```python
from build123d import *

# Parameters (mm, degrees)
CYLINDER003_R     = 2
CYLINDER003_DEPTH = 10
CYLINDER001_R     = 2
CYLINDER001_DEPTH = 10
SKETCH037_W       = 7.5
SKETCH037_H       = 7.5
EXTRUDE045_DEPTH  = 10
SKETCH005_R       = 1.3
EXTRUDE003_DEPTH  = 20
EXTRUDE039_DEPTH  = 4
EXTRUDE042_DEPTH  = 0.8
EXTRUDE002_DEPTH  = 6
EXTRUDE037_DEPTH  = 2


with BuildPart() as shutter_cable001:
    # Cylinder003 → Cylinder003 (new body)
    with BuildSketch(Plane(origin=(19.5, 0, 24.5), x_dir=(1, 0, 0), z_dir=(0, 0, 1))):
        Circle(CYLINDER003_R)
    extrude(amount=CYLINDER003_DEPTH)


with BuildPart() as battery_cable:
    # Cylinder001 → Cylinder001 (new body)
    with BuildSketch(Plane(origin=(-70.5, 0, 12), x_dir=(0, 0, 1), z_dir=(-1, 0, 0))):
        Circle(CYLINDER001_R)
    extrude(amount=CYLINDER001_DEPTH)


with BuildPart() as common_sub:
    # Sketch037 → Extrude045 (new body)
    with BuildSketch(Plane.YZ.offset(35)):
        with Locations((0, 12)):
            Rectangle(SKETCH037_W, SKETCH037_H)
    extrude(amount=EXTRUDE045_DEPTH)


with BuildPart() as common_sub_1:
    # Extrude045 placement: moved
    add(common_sub.part.moved(Location((-9.5, 0, 0))))

    # Fusion033: union shutter cable001, battery cable
    add(shutter_cable001.part)
    add(battery_cable.part)


with BuildPart() as sweep001:
    # Sweep001: sweep along a path in Sketch034
    with BuildLine(Plane.XZ.offset(10)) as sweep001_path:
        Line((32, 12), (32, 26.4))
        ThreePointArc((32, 26.4), (30.652691, 29.652691), (27.4, 31))
        Line((27.4, 31), (-39.9, 31))
    # Sketch035 → Sweep001 (sweep)
    with BuildSketch(Plane.YZ):
        Polygon((5.3, 29.4), (3.7, 31), (3.7, 32), (6, 32), (6, 29.4), align=None)
    sweep(path=sweep001_path.line)


with BuildPart() as fusion030:
    # Sketch005 → Extrude003 (new body)
    with BuildSketch(Plane.XZ.offset(5)):
        with Locations((27.4, 26.4)):
            Circle(SKETCH005_R)
    extrude(amount=-EXTRUDE003_DEPTH)


with BuildPart() as fusion030_1:
    # Extrude003 placement: moved
    add(fusion030.part.moved(Location((0, -4, 0))))

    # Fusion030: union Sweep001
    add(sweep001.part)


with BuildPart() as top003:
    # Sketch028 → Extrude039 (new body)
    with BuildSketch(Plane.XZ.offset(10)):
        with BuildLine():
            ThreePointArc((32, 26.4), (30.652691, 29.652691), (27.4, 31))
            Line((27.4, 31), (-39.9, 31))
            Line((-39.9, 31), (-39.9, 29))
            Line((-39.9, 29), (27.4, 29))
            ThreePointArc((30, 26.4), (29.238478, 28.238478), (27.4, 29))
            Line((30, 12), (30, 26.4))
            Line((32, 12), (30, 12))
            Line((32, 26.4), (32, 12))
        make_face()
    extrude(amount=EXTRUDE039_DEPTH)


with BuildPart() as top003_1:
    # Extrude039 placement: moved
    add(top003.part.moved(Location((0, 14.5, 0))))


with BuildPart() as top002:
    # Sketch031 → Extrude042 (new body)
    with BuildSketch(Plane.XZ.offset(10)):
        with BuildLine():
            ThreePointArc((32, 26.4), (30.652691, 29.652691), (27.4, 31))
            Line((27.4, 31), (-39.9, 31))
            Line((-39.9, 31), (-39.9, 12))
            Line((-39.9, 12), (32, 12))
            Line((32, 26.4), (32, 12))
        make_face()
    extrude(amount=EXTRUDE042_DEPTH)


with BuildPart() as top002_1:
    # Extrude042 placement: moved
    add(top002.part.moved(Location((0, 15.3, 0))))


with BuildPart() as screw_hole_top:
    # Sketch004 → Extrude002 (new body)
    with BuildSketch(Plane.XZ.offset(10)):
        with BuildLine():
            ThreePointArc((25.36776, 29), (25.066548, 24.066548), (30, 24.36776))
            Line((30, 24.36776), (30, 26.4))
            ThreePointArc((30, 26.4), (29.238478, 28.238478), (27.4, 29))
            Line((25.36776, 29), (27.4, 29))
        make_face()
    extrude(amount=-EXTRUDE002_DEPTH)


with BuildPart() as screw_hole_top_1:
    # Extrude002 placement: moved
    add(screw_hole_top.part.moved(Location((0, 8.5, 0))))


with BuildPart() as top:
    # Sketch029 → Extrude037 (new body)
    with BuildSketch(Plane.XZ.offset(10)):
        with BuildLine():
            ThreePointArc((30.9, 26.4), (29.874874, 28.874874), (27.4, 29.9))
            Line((27.4, 29.9), (-22.5, 29.9))
            Line((-22.5, 29.9), (-22.5, 29))
            Line((-22.5, 29), (27.4, 29))
            ThreePointArc((30, 26.4), (29.238478, 28.238478), (27.4, 29))
            Line((30, 12), (30, 26.4))
            Line((30.9, 12), (30, 12))
            Line((30.9, 26.4), (30.9, 12))
        make_face()
    extrude(amount=EXTRUDE037_DEPTH)


with BuildPart() as top_1:
    # Extrude037 placement: moved
    add(top.part.moved(Location((0, 10.5, 0))))

    # Fusion028: union top003, top002, screw hole top
    add(top003_1.part)
    add(top002_1.part)
    add(screw_hole_top_1.part)

    # Cut024: cut Fusion030
    add(fusion030_1.part, mode=Mode.SUBTRACT)


with BuildPart() as part_mirroring:
    # Part__Mirroring: instance of top
    add(top_1.part.mirror(Plane(origin=(0, 0, 12), x_dir=(0, 1, 0), z_dir=(0, 0, 1))))


with BuildPart() as part_mirroring002:
    # Part__Mirroring002: instance of Part__Mirroring
    add(part_mirroring.part.mirror(Plane(origin=(-22.5, 1, 0), x_dir=(0, -1, 0), z_dir=(1, 0, 0))))


with BuildPart() as top007:
    # Part__Mirroring003: instance of top
    add(top_1.part.mirror(Plane(origin=(-22.5, 0, 0), x_dir=(0, -1, 0), z_dir=(1, 0, 0))))

    # Fusion032: union top, Part__Mirroring, Part__Mirroring002
    add(top_1.part)
    add(part_mirroring.part)
    add(part_mirroring002.part)

    # Cut025: cut common sub
    add(common_sub_1.part, mode=Mode.SUBTRACT)


solid = top007.part
```
Can you work these out from the model? Positions are in its coordinate system, mm. A direction names the side the tool comes from. Coordinates: 2 decimals unless noted, no trailing zeros. Write each loop counter-clockwise with the first axis right and the second up, starting at its lowest first coordinate (ties: lowest second). Pieces come first, ordered by that corner, then holes. Notation, with made-up numbers: M 60.5,21 L 78.5,21 A14 cw 78.5,45 Z; hole C 50,1.5 d7. An arc over 180 degrees is marked long. Write item = value, one per line. Start each with the question number.
Q1. If I drill on L1, parallel to Z at x = -72.4, y = 3.5; L2, parallel to Z at x = -65.5, y = -1; L3, parallel to X at y = 1.5, z = 25.5, over which ranges is the centre line in solid material (lowest first)? Write a range as [from, to].
Q2. I'm going to push flat-ended pins straight in: pin 1 (0.6 mm diameter, centred on y = -1, z = 21.5, fed in from -X); pin 2 (0.6 mm diameter, centred on x = 30.5, y = 2, fed in from -Z); pin 3 (1 mm diameter, centred on x = -12, y = 4.5, fed in from +Z). Where does each tip first touch, or does it pass through?
Q3. If we section it at C-C, the plane z = 12: Write out the boundary of the cut face in (x, y), then the cut area to 3 significant figures.
Q4. If we section it at B-B, the plane x = -58: Write out the boundary of the cut face in (y, z), then the cut area to 3 significant figures.
Q5. On a 3-axis mill with a long thin cutter (end or side, diameter ignored), from which of +Z, -Z, +X, -X, +Y, -Y can I reach the whole of each face in a straight line? I mean faces 1 (the face through (-74.9, -0.49, 28.85)), 2 (the face through (-75.9, 0, 20)), 3 (the face through (-22, 2, -5)). Say none if no direction works.
Q6. Thinking about a two-plate mould opening in Z: for faces 4 (the face through (31, 3.75, 12)), 5 (the face through (-71.1, 1.85, -2.46)), 6 (the face through (-23, 2, -7)), 7 (the face through (30.9, 0, 3)), which applies, released by +Z, released by -Z, zero draft, split by the parting line, or undercut?
Q7. If we section it at A-A, the plane z = 21.5: Write out the boundary of the cut face in (x, y), then the cut area to 3 significant figures.
Check sheet entries:
q1.L1 = [-7, -3.7], [-1.1, 0.9], [23.1, 25.1], [27.7, 31]
q1.L2 = [-5.9, -5], [29, 29.9]
q1.L3 = [-77, -73.34], [-71.46, -69.23], [24.23, 26.46], [28.34, 32]
q2.pin_1 = -75.9
q2.pin_2 = -6.05
q2.pin_3 = 30.7
q3.outline = M -77,2 L -75,2 L -75,4.5 L 30,4.5 L 30,3.75 L 31.95,3.75 L 30.4,5.3 L -75.4,5.3 L -77,3.7 Z
q3.area = 91.1 mm²
q4.outline = M -1.5,-5.9 L 0.5,-5.9 L 0.5,-7 L 3.7,-7 L 5.3,-5.4 L 5.3,29.4 L 3.7,31 L 0.5,31 L 0.5,29.9 L -1.5,29.9 L -1.5,29 L 4.5,29 L 4.5,-5 L -1.5,-5 Z
q4.area = 47.4 mm²
q5.face_1 = +Z, -X, -Y
q5.face_2 = +Z, -Z, -X, -Y
q5.face_3 = -Y
q6.face_4 = undercut
q6.face_5 = undercut
q6.face_6 = released by -Z
q6.face_7 = zero draft
q7.outline = M -77,0.5 L -75.9,0.5 L -75.9,-1.5 L -75,-1.5 L -75,4.5 L 30,4.5 L 30,-1.5 L 30.9,-1.5 L 30.9,0.5 L 32,0.5 L 32,3.7 L 30.4,5.3 L -75.4,5.3 L -77,3.7 Z
q7.area = 104 mm²
